The model under review builds one solid part; all positions refer to its coordinate system, in mm. Give positions to 0.01 mm unless a question says otherwise; leave off trailing zeros. Order: outer loops, then holes, each group sorted by start corner. A loop starts at its lowest first (then second) coordinate and runs counter-clockwise, first axis right, second up. Notation, with made-up numbers: (-23.5, 27.5) - (-0.5, 27.5) arc R23 cw to (-0.5, 64.5) - close; hole circle Ø2 at (3.25, -6). An arc over 180 degrees is marked (long way). Write item = value, one per line. Start each with the question number.
1. We need section A-A, the plane y = 26. Give the boundary of the cut face in (x, z).
2. We need section D-D, the plane x = 17.5. Give the boundary of the cut face in (y, z).
3. We need section B-B, the plane x = -6. Give the boundary of the cut face in (y, z), and give its area (3 significant figures).
4. We need section C-C, the plane y = -28. Give the boundary of the cut face in (x, z), and give its area (3 significant figures).
5. Wall thickness on probe 1 along Y at (x, z) = (47.5, 1.15); probe 2 along Y at (x, z) = (61, 1.7); probe 3 along Y at (x, z) = (16, 0.25): over which ranges is each line inside the solid? List them lowest first.
6. For P1, Ø12, axis at x = 28.5, y = -27, coming from the -Z side; P2, Ø0.9, axis at x = 71, z = 2, coming from the -Y side; P3, Ø0.9, axis at y = -1.5, z = 1.5, coming from the -X side; P4, Ø0.9, axis at x = -68.5, z = 1, coming from the -Y side, all flat-tipped, find the tip position at first contact; note any pin that passes through.
from build123d import *

# Parameters (mm, degrees)
SKETCH_1_W              = 180
SKETCH_1_H              = 72
EXTRUDE_1_DEPTH         = 3
HOLE_WIZARD_4_2_4_2_1_D = 4.2
CUT_EXTRUDE_2_DEPTH     = 97.979379251
CUT_EXTRUDE_3_DEPTH     = 97.979379251


with BuildPart() as part:
    # 草图1 → 凸台-拉伸1 (new body)
    with BuildSketch(Plane.XY):
        Rectangle(SKETCH_1_W, SKETCH_1_H)
    extrude(amount=EXTRUDE_1_DEPTH)

    # Ø4.2 (4.2) 直径孔1 (through all)
    with Locations(Plane(origin=(-62.5, 26, 3), x_dir=(1, 0, 0), z_dir=(0, 0, 1))):
        with Locations((0, 0), (30, 0), (15, -29), (15, -54), (110, -54), (110, -29), (125, 0), (95, 0)):
            Hole(HOLE_WIZARD_4_2_4_2_1_D / 2)

    # 草图8 → 切除-拉伸2 (cut, through all)
    with BuildSketch(Plane(origin=(0, 0, 0), x_dir=(-1, 0, 0), z_dir=(0, 0, -1))):
        Polygon((-90, 16), (-57.5, -36), (-90, -36), align=None)
        Polygon((90, -36), (90, 16), (57.5, -36), align=None)
    extrude(amount=-CUT_EXTRUDE_2_DEPTH, mode=Mode.SUBTRACT)

    # 草图6 → 切除-拉伸3 (cut, through all)
    with BuildSketch(Plane(origin=(0, 0, 0), x_dir=(-1, 0, 0), z_dir=(0, 0, -1))):
        with BuildLine():
            Line((57.5, 14), (57.5, -13.932037736))
            ThreePointArc((57.5, -13.932037736), (58.948634974, -15.854535228), (61.195996608, -14.992035616))
            Line((61.195996608, -14.992035616), (78.653520193, 12.94000212))
            ThreePointArc((78.653520193, 12.94000212), (78.706808547, 14.969537065), (76.957523585, 16))
            Line((76.957523585, 16), (59.5, 16))
            ThreePointArc((59.5, 16), (58.085786438, 15.414213562), (57.5, 14))
        make_face()
        with BuildLine():
            Line((-76.957523585, 16), (-59.5, 16))
            ThreePointArc((-59.5, 16), (-58.085786438, 15.414213562), (-57.5, 14))
            Line((-57.5, 14), (-57.5, -13.932037736))
            ThreePointArc((-57.5, -13.932037736), (-58.948634974, -15.854535228), (-61.195996608, -14.992035616))
            Line((-61.195996608, -14.992035616), (-78.653520193, 12.94000212))
            ThreePointArc((-78.653520193, 12.94000212), (-78.706808547, 14.969537065), (-76.957523585, 16))
        make_face()
        with BuildLine():
            Line((-23.394059646, 16), (23.394059646, 16))
            ThreePointArc((23.394059646, 16), (25.347497325, 14.429046887), (24.232176, 12.184081231))
            Line((24.232176, 12.184081231), (0.838116355, 1.386822933))
            ThreePointArc((0.838116355, 1.386822933), (0, 1.202741702), (-0.838116355, 1.386822933))
            Line((-0.838116355, 1.386822933), (-24.232176, 12.184081231))
            ThreePointArc((-24.232176, 12.184081231), (-25.347497325, 14.429046887), (-23.394059646, 16))
        make_face()
        with BuildLine():
            Line((-37.5, 8.181873683), (-37.5, -13.181873683))
            ThreePointArc((-37.5, -13.181873683), (-36.577907067, -14.866544676), (-34.661883645, -14.997792452))
            Line((-34.661883645, -14.997792452), (-11.517824, -4.315918769))
            ThreePointArc((-11.517824, -4.315918769), (-10.355940354, -2.5), (-11.517824, -0.684081231))
            Line((-11.517824, -0.684081231), (-34.661883645, 9.997792452))
            ThreePointArc((-34.661883645, 9.997792452), (-36.577907067, 9.866544676), (-37.5, 8.181873683))
        make_face()
        with BuildLine():
            Line((-23.394059646, -21), (23.394059646, -21))
            ThreePointArc((23.394059646, -21), (25.347497325, -19.429046887), (24.232176, -17.184081231))
            Line((24.232176, -17.184081231), (0.838116355, -6.386822933))
            ThreePointArc((0.838116355, -6.386822933), (0, -6.202741702), (-0.838116355, -6.386822933))
            Line((-0.838116355, -6.386822933), (-24.232176, -17.184081231))
            ThreePointArc((-24.232176, -17.184081231), (-25.347497325, -19.429046887), (-23.394059646, -21))
        make_face()
        with BuildLine():
            Line((37.5, 8.181873683), (37.5, -13.181873683))
            ThreePointArc((37.5, -13.181873683), (36.577907067, -14.866544676), (34.661883645, -14.997792452))
            Line((34.661883645, -14.997792452), (11.517824, -4.315918769))
            ThreePointArc((11.517824, -4.315918769), (10.355940354, -2.5), (11.517824, -0.684081231))
            Line((11.517824, -0.684081231), (34.661883645, 9.997792452))
            ThreePointArc((34.661883645, 9.997792452), (36.577907067, 9.866544676), (37.5, 8.181873683))
        make_face()
    extrude(amount=-CUT_EXTRUDE_3_DEPTH, mode=Mode.SUBTRACT)


solid = part.part
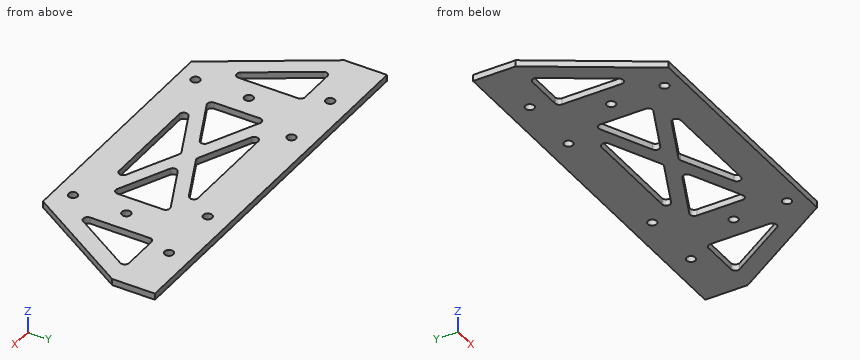
Model answer:
q1.outline = (-90, 0) - (-64.6, 0) - (-64.6, 3) - (-90, 3) - close; (-60.4, 0) - (-34.6, 0) - (-34.6, 3) - (-60.4, 3) - close; (-30.4, 0) - (30.4, 0) - (30.4, 3) - (-30.4, 3) - close; (34.6, 0) - (60.4, 0) - (60.4, 3) - (34.6, 3) - close; (64.6, 0) - (90, 0) - (90, 3) - (64.6, 3) - close
q2.outline = (-36, 0) - (-21, 0) - (-21, 3) - (-36, 3) - close; (-14.08, 0) - (-7.08, 0) - (-7.08, 3) - (-14.08, 3) - close; (2.08, 0) - (9.08, 0) - (9.08, 3) - (2.08, 3) - close; (16, 0) - (36, 0) - (36, 3) - (16, 3) - close
q3.outline = (-36, 0) - (-21, 0) - (-21, 3) - (-36, 3) - close; (-8.77, 0) - (3.77, 0) - (3.77, 3) - (-8.77, 3) - close; (16, 0) - (36, 0) - (36, 3) - (16, 3) - close
q3.area = 143 mm2
q4.outline = (-62.5, 0) - (-49.6, 0) - (-49.6, 3) - (-62.5, 3) - close; (-45.4, 0) - (45.4, 0) - (45.4, 3) - (-45.4, 3) - close; (49.6, 0) - (62.5, 0) - (62.5, 3) - (49.6, 3) - close
q4.area = 350 mm2
q5.probe_1 = -36 to -30.1, -25.9 to -5.1, -0.9 to 36
q5.probe_2 = -30.4 to -15.25, 16 to 24.53, 27.47 to 36
q5.probe_3 = -36 to -21, -13.38 to -6.38, 1.38 to 8.38, 16 to 36
q6.P1 = 0
q6.P2 = -15.12
q6.P3 = -79.34
q6.P4 = -19.12
